Model file for the job. Use its own axes, mm. Face numbers are marked on the shaded views. A direction names the side the tool comes from. Round coordinates to 2 decimals unless told otherwise and drop trailing zeros. Order: outer loops, then holes, each group sorted by start corner. A loop starts at its lowest first (then second) coordinate and runs counter-clockwise, first axis right, second up. Notation, with made-up numbers: (-36.75, 35) - (6.25, 35) arc R28 cw to (6.25, 60) - close; hole circle Ø5 at (-31, -10). An arc over 180 degrees is marked (long way). Use one line per item in the form item = value.
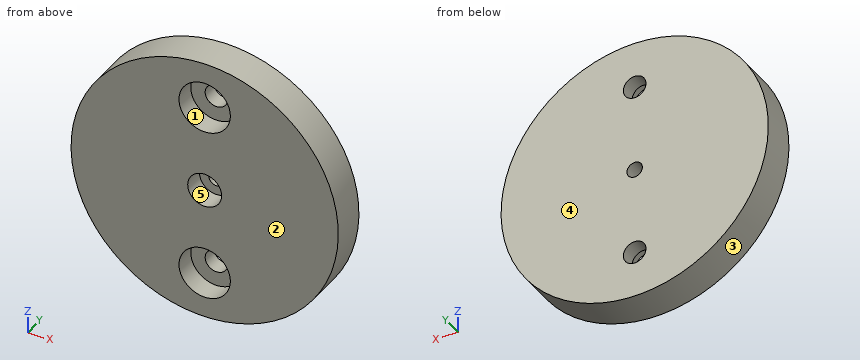
from build123d import *

# Parameters (mm, degrees)
SKETCH1_R           = 13
SKETCH1_R_2         = 1.65
SKETCH1_R_3         = 2.5
BOSS_EXTRUDE1_DEPTH = 2
SKETCH2_R           = 13
SKETCH2_R_2         = 0.75
SKETCH2_R_3         = 1.1
BOSS_EXTRUDE2_DEPTH = 1.5


with BuildPart() as part:
    # Sketch1 → Boss-Extrude1 (new body)
    with BuildSketch(Plane(origin=(0, 0, 0), x_dir=(1, 0, 0), z_dir=(0, 1, 0))):
        with Locations(Location((0, 0, 0), (0, 0, 270))):
            Circle(SKETCH1_R)
        with Locations(Location((0, 0, 0), (0, 0, 270))):
            Circle(SKETCH1_R_2, mode=Mode.SUBTRACT)
        with Locations(Location((0, 8.5, 0), (0, 0, 270))):
            Circle(SKETCH1_R_3, mode=Mode.SUBTRACT)
        with Locations(Location((0, -8.5, 0), (0, 0, 270))):
            Circle(SKETCH1_R_3, mode=Mode.SUBTRACT)
    extrude(amount=BOSS_EXTRUDE1_DEPTH)

    # Sketch2 → Boss-Extrude2 (add)
    with BuildSketch(Plane(origin=(0, 2, 0), x_dir=(1, 0, 0), z_dir=(0, 1, 0))):
        with Locations(Location((0, 0, 0), (0, 0, 270))):
            Circle(SKETCH2_R)
        with Locations(Location((0, 0, 0), (0, 0, 270))):
            Circle(SKETCH2_R_2, mode=Mode.SUBTRACT)
        with Locations(Location((0, 8.5, 0), (0, 0, 270))):
            Circle(SKETCH2_R_3, mode=Mode.SUBTRACT)
        with Locations(Location((0, -8.5, 0), (0, 0, 270))):
            Circle(SKETCH2_R_3, mode=Mode.SUBTRACT)
    extrude(amount=BOSS_EXTRUDE2_DEPTH)


solid = part.part
(1) Slice it at C-C on y = 3.1. Give the cut face in (x, z).
Report:
outline = circle Ø26 at (0, 0); hole circle Ø2.2 at (0, -8.5); hole circle Ø2.2 at (0, 8.5); hole circle Ø1.5 at (0, 0)
(2) Slice it at B-B on x = 0. Give the cut face in (y, z), then the cut area to 4 significant figures.
Report:
outline = (0, -13) - (3.5, -13) - (3.5, -9.6) - (2, -9.6) - (2, -11) - (0, -11) - close; (0, -6) - (2, -6) - (2, -7.4) - (3.5, -7.4) - (3.5, -0.75) - (2, -0.75) - (2, -1.65) - (0, -1.65) - close; (0, 1.65) - (2, 1.65) - (2, 0.75) - (3.5, 0.75) - (3.5, 7.4) - (2, 7.4) - (2, 6) - (0, 6) - close; (0, 11) - (2, 11) - (2, 9.6) - (3.5, 9.6) - (3.5, 13) - (0, 13) - close
area = 55.55 mm2
(3) Slice it at D-D on z = 8.5. Give the cut face in (x, y), then the cut area to 3 significant figures.
Report:
outline = (-9.84, 0) - (-2.5, 0) - (-2.5, 2) - (-1.1, 2) - (-1.1, 3.5) - (-9.84, 3.5) - close; (1.1, 2) - (2.5, 2) - (2.5, 0) - (9.84, 0) - (9.84, 3.5) - (1.1, 3.5) - close
area = 55.6 mm2
(4) Probe probe 1 along X at (y, z) = (2.65, -8.5); probe 2 along X at (y, z) = (2.45, -9.25); probe 3 along X at (y, z) = (1.15, -5.5). List the from-to ranges inside material, lowest first. Write a range as [from, to].
Report:
probe_1 = [-9.84, -1.1], [1.1, 9.84]
probe_2 = [-9.13, -0.8], [0.8, 9.13]
probe_3 = [-11.78, 11.78]
(5) Pin check, flat tips, straight feed: pin 1 (2 mm diameter, centred on y = 1, z = -5.5, fed in from +X); pin 2 (1.3 mm diameter, centred on x = 0, z = -8.5, fed in from -Y); pin 3 (1.6 mm diameter, centred on x = -0.5, z = 0.5, fed in from -Y); pin 4 (1 mm diameter, centred on y = 2.5, z = 2.5, fed in from -X). Stop position of each tip, or through.
Report:
pin_1 = 12.2
pin_2 = through
pin_3 = 2
pin_4 = -12.85
(6) Tool access for the marked faces 1 and 2: list every direction of +Z, -Z, +X, -X, +Y, -Y with a clear straight run to the whole face (end or side of a thin tool).
Report:
face_1 = -Y
face_2 = +Z, -Z, +X, -X, -Y
(7) Slice it at A-A on z = 0. Give the cut face in (x, y).
Report:
outline = (-13, 0) - (-1.65, 0) - (-1.65, 2) - (-0.75, 2) - (-0.75, 3.5) - (-13, 3.5) - close; (0.75, 2) - (1.65, 2) - (1.65, 0) - (13, 0) - (13, 3.5) - (0.75, 3.5) - close
(8) Pull direction Z, two halves, no side cores. Call the marked faces 3, 4 and 5: released by +Z, released by -Z, zero draft, split by the parting line, or undercut.
Report:
face_3 = split by the parting line
face_4 = zero draft
face_5 = undercut
